Here's how the part is built. I have some questions about the finished solid (model axes, mm). A direction names the side the tool comes from. Coordinates: 2 decimals unless noted, no trailing zeros. Loops run counter-clockwise (first coordinate to the right, second up) from the corner with the lowest first, then second, coordinate; pieces in that order, holes last. Notation, with made-up numbers: (-30.5, 70.5) -> (22.5, 70.5) arc R33 cw to (22.5, 105.5) -> close; hole circle Ø9 at (0, -27). An arc over 180 degrees is marked (long way). Answer as a JSON object with one key per item and string values. Group by question number.
1) I want a section at A-A (y = 11.5). Write out the boundary of the cut face in (x, z), then the cut area to 3 significant figures.
2) I want a section at D-D (x = -24.25). Write out the boundary of the cut face in (y, z).
3) I need wall thicknesses on probe 1 along Y at (x, z) = (24.25, -26.5); probe 2 along X at (y, z) = (15, -28.5); probe 3 along X at (y, z) = (15, -26.5). Which ranges of each line are inside material? Lowest first, please. Write a range as [from, to].
4) I want a section at C-C (y = 5). Write out the boundary of the cut face in (x, z).
5) I want a section at B-B (z = -32). Count the separate pieces of the cut face and the enclosed holes in it, then the cut area to 3 significant figures.
6) I'm going to push flat-ended pins straight in: pin 1 (8 mm diameter, centred on x = -23, y = 13.5, fed in from -Z); pin 2 (8 mm diameter, centred on y = 1.5, z = -11.5, fed in from +X); pin 3 (15.5 mm diameter, centred on x = -25, z = -15, fed in from +Y). Where does each tip first touch, or does it pass through?
7) Which directions (+Z, -Z, +X, -X, +Y, -Y) give clear straight access to the entire face, cutting with the end or side of a thin tool? Please do faces 4 (the flat face through (16.5, -1, -23)), 5 (the flat face through (24, 10, -23.214)), 6 (the flat face through (24, 9, -33.214)), 7 (the flat face through (24, 6.5, -28)).
8) If we mould it in two halves opening along X, with no side actions, what happens to faces 1 (the flat face through (-24, 19, -28)), 2 (the flat face through (-16.5, -1, -23)), 3 (the flat face through (-30.75, -1, -32))? For each: +X half, -X half, draft (parallel to the pull), parting line (faces both ways), or undercut.
```python
from build123d import *

# Parameters (mm, degrees)
BOSS_EXTRUDE1_DEPTH = 4.5
SKETCH2_W           = 33
SKETCH2_H           = 47
CUT_EXTRUDE1_DEPTH  = 2.25
BOSS_EXTRUDE2_DEPTH = 2
BOSS_EXTRUDE3_DEPTH = 19
CHAMFER1_SIZE       = 2
CHAMFER2_SIZE       = 2
CUT_EXTRUDE2_REACH  = 45.27


with BuildPart() as part:
    # Sketch1 → Boss-Extrude1 (new body)
    with BuildSketch(Plane(origin=(0, 0, 0), x_dir=(1, 0, 0), z_dir=(0, 1, 0))):
        Polygon((21.25, 0), (-21.25, 0), (-30.75, 27), (-30.75, 37), (-20.75, 47), (20.75, 47), (30.75, 37), (30.75, 27), align=None)
    extrude(amount=-BOSS_EXTRUDE1_DEPTH)

    # Sketch2 → Cut-Extrude1 (cut)
    with BuildSketch(Plane(origin=(0, 0, 0), x_dir=(1, 0, 0), z_dir=(0, 1, 0))):
        with Locations((0, 23.5)):
            Rectangle(SKETCH2_W, SKETCH2_H)
    extrude(amount=-CUT_EXTRUDE1_DEPTH, mode=Mode.SUBTRACT)

    # Sketch3 → Boss-Extrude2 (add)
    with BuildSketch(Plane(origin=(0, 0, 0), x_dir=(1, 0, 0), z_dir=(0, 1, 0))):
        Polygon((-21.25, 0), (-16.5, 0), (-16.5, 2.5), (-19.479394115, 2.5), (-28.25, 27.426985148), (-28.25, 35.964466094), (-19.714466094, 44.5), (-16.5, 44.5), (-16.5, 47), (-20.75, 47), (-30.75, 37), (-30.75, 27), align=None)
        Polygon((16.5, 0), (21.25, 0), (30.75, 27), (30.75, 37), (20.75, 47), (16.5, 47), (16.5, 44.5), (19.714466094, 44.5), (28.25, 35.964466094), (28.25, 27.426985148), (19.479394115, 2.5), (16.5, 2.5), align=None)
    extrude(amount=BOSS_EXTRUDE2_DEPTH)

    # Sketch4 → Boss-Extrude3 (add)
    with BuildSketch(Plane(origin=(0, 0, 0), x_dir=(1, 0, 0), z_dir=(0, 1, 0))):
        Polygon((-20.25, 33.214466094), (-20.25, 23.214466094), (-26.76781737, 23.214466094), (-28.25, 27.426985148), (-28.25, 33.214466094), align=None)
        Polygon((20.25, 23.214466094), (20.25, 33.214466094), (28.25, 33.214466094), (28.25, 27.426985148), (26.76781737, 23.214466094), align=None)
    extrude(amount=BOSS_EXTRUDE3_DEPTH)

    # Chamfer1
    chamfer1_edges = [part.edges().sort_by_distance(p)[0] for p in [
        (-27.508908685, 2, -25.320725621),
        (28.25, 2, -30.320725621),
        (-28.25, 2, -30.320725621),
        (27.508908685, 2, -25.320725621),
    ]]
    chamfer(chamfer1_edges, length=CHAMFER1_SIZE)

    # Chamfer2
    chamfer2_edges = [part.edges().sort_by_distance(p)[0] for p in [
        (23.508908685, 0, -23.214466094),
        (-23.508908685, 0, -23.214466094),
    ]]
    chamfer(chamfer2_edges, length=CHAMFER2_SIZE)

    # Sketch5 → Cut-Extrude2 (cut, up to next)
    with BuildSketch(Plane.XY.offset(-23.214466094), mode=Mode.PRIVATE) as cut_extrude2_sk1:
        with BuildLine():
            Line((-24.949461487, 16.5), (-25.399066665, 15.964181415))
            ThreePointArc((-25.399066665, 15.964181415), (-24.25, 13.5), (-23.100933335, 15.964181415))
            Line((-23.100933335, 15.964181415), (-23.550538513, 16.5))
            Line((-23.550538513, 16.5), (-24.949461487, 16.5))
        make_face()
    cut_extrude2_tool1 = extrude(cut_extrude2_sk1.sketch, amount=-CUT_EXTRUDE2_REACH, mode=Mode.PRIVATE) & part.part
    # Sketch5 → Cut-Extrude2 (cut, up to next)
    with BuildSketch(Plane.XY.offset(-23.214466094), mode=Mode.PRIVATE) as cut_extrude2_sk2:
        with BuildLine():
            Line((-23.100933335, 5.964181415), (-23.550538513, 6.5))
            Line((-23.550538513, 6.5), (-24.949461487, 6.5))
            Line((-24.949461487, 6.5), (-25.399066665, 5.964181415))
            ThreePointArc((-25.399066665, 5.964181415), (-24.25, 3.5), (-23.100933335, 5.964181415))
        make_face()
    cut_extrude2_tool2 = extrude(cut_extrude2_sk2.sketch, amount=-CUT_EXTRUDE2_REACH, mode=Mode.PRIVATE) & part.part
    # Sketch5 → Cut-Extrude2 (cut, up to next)
    with BuildSketch(Plane.XY.offset(-23.214466094), mode=Mode.PRIVATE) as cut_extrude2_sk3:
        with BuildLine():
            Line((23.100933335, 5.964181415), (23.550538513, 6.5))
            Line((23.550538513, 6.5), (24.949461487, 6.5))
            Line((24.949461487, 6.5), (25.399066665, 5.964181415))
            ThreePointArc((25.399066665, 5.964181415), (24.25, 3.5), (23.100933335, 5.964181415))
        make_face()
    cut_extrude2_tool3 = extrude(cut_extrude2_sk3.sketch, amount=-CUT_EXTRUDE2_REACH, mode=Mode.PRIVATE) & part.part
    # Sketch5 → Cut-Extrude2 (cut, up to next)
    with BuildSketch(Plane.XY.offset(-23.214466094), mode=Mode.PRIVATE) as cut_extrude2_sk4:
        with BuildLine():
            Line((24.949461487, 16.5), (25.399066665, 15.964181415))
            ThreePointArc((25.399066665, 15.964181415), (24.25, 13.5), (23.100933335, 15.964181415))
            Line((23.100933335, 15.964181415), (23.550538513, 16.5))
            Line((23.550538513, 16.5), (24.949461487, 16.5))
        make_face()
    cut_extrude2_tool4 = extrude(cut_extrude2_sk4.sketch, amount=-CUT_EXTRUDE2_REACH, mode=Mode.PRIVATE) & part.part
    add(cut_extrude2_tool1.solids().sort_by_distance((-24.25, 15.026014, -23.214466))[0], mode=Mode.SUBTRACT)
    add(cut_extrude2_tool2.solids().sort_by_distance((-24.25, 5.026014, -23.214466))[0], mode=Mode.SUBTRACT)
    add(cut_extrude2_tool3.solids().sort_by_distance((24.25, 5.026014, -23.214466))[0], mode=Mode.SUBTRACT)
    add(cut_extrude2_tool4.solids().sort_by_distance((24.25, 15.026014, -23.214466))[0], mode=Mode.SUBTRACT)


solid = part.part
```
Determined:
{
 "1": {"outline": "(-28.25, -33.21) -> (-20.25, -33.21) -> (-20.25, -23.21) -> (-26.77, -23.21) -> (-28.25, -27.43) -> close; (20.25, -33.21) -> (28.25, -33.21) -> (28.25, -27.43) -> (26.77, -23.21) -> (20.25, -23.21) -> close", "area": "154 mm^2"},
 "2": {"outline": "(-4.5, -43.5) -> (2, -43.5) -> (2, -39.96) -> (0, -39.96) -> (0, -33.21) -> (3.5, -33.21) -> (3.5, -23.21) -> (2, -23.21) -> (0, -21.21) -> (0, -16.06) -> (2, -16.06) -> (2, -8.53) -> (-4.5, -8.53) -> close; (6.5, -33.21) -> (13.5, -33.21) -> (13.5, -23.21) -> (6.5, -23.21) -> close; (16.5, -33.21) -> (19, -33.21) -> (19, -23.21) -> (16.5, -23.21) -> close"},
 "3": {"probe 1": "[-4.5, 3.5], [6.5, 13.5], [16.5, 19]", "probe 2": "[-28.25, -25.75], [-22.75, -20.25], [20.25, 22.75], [25.75, 28.25]", "probe 3": "[-27.92, -25.75], [-22.75, -20.25], [20.25, 22.75], [25.75, 27.92]"},
 "4": {"outline": "(-28.25, -33.21) -> (-25.75, -33.21) -> (-25.75, -23.21) -> (-26.77, -23.21) -> (-28.25, -27.43) -> close; (-22.75, -33.21) -> (-20.25, -33.21) -> (-20.25, -23.21) -> (-22.75, -23.21) -> close; (20.25, -33.21) -> (22.75, -33.21) -> (22.75, -23.21) -> (20.25, -23.21) -> close; (25.75, -33.21) -> (28.25, -33.21) -> (28.25, -27.43) -> (26.77, -23.21) -> (25.75, -23.21) -> close"},
 "5": {"separate pieces": "1", "enclosed holes": "4", "area": "492 mm^2"},
 "6": {"pin 1": "z = -33.21", "pin 2": "x = 26.7", "pin 3": "y = 2"},
 "7": {"face 4": "+Z, -Z, +Y", "face 5": "+Z, +X, -X, +Y", "face 6": "+Y", "face 7": "+Z, -Z"},
 "8": {"face 1": "draft", "face 2": "undercut", "face 3": "-X half"}
}
